```python
from build123d import *

# Parameters (mm, degrees)
ESQUISSE1_W             = 54.1
ESQUISSE1_H             = 54.4
BOSS_EXTRU_1_DEPTH      = 19
ESQUISSE2_W             = 20
ESQUISSE2_H             = 12
BOSS_EXTRU_2_DEPTH      = 15
ESQUISSE3_W             = 9
ESQUISSE3_H             = 18
BOSS_EXTRU_3_DEPTH      = 5
ESQUISSE4_R             = 1.5
ENL_V_MAT_EXTRU_1_DEPTH = 81.387623426


with BuildPart() as part:
    # Esquisse1 → Boss.-Extru.1 (new body)
    with BuildSketch(Plane(origin=(0, 0, 0), x_dir=(1, 0, 0), z_dir=(0, 1, 0))):
        with Locations((27.05, 27.2)):
            Rectangle(ESQUISSE1_W, ESQUISSE1_H)
    extrude(amount=BOSS_EXTRU_1_DEPTH)

    # Esquisse2 → Boss.-Extru.2 (add)
    with BuildSketch(Plane.XZ):
        with Locations((27, -28.4)):
            Rectangle(ESQUISSE2_W, ESQUISSE2_H)
    extrude(amount=BOSS_EXTRU_2_DEPTH)

    # Esquisse3 → Boss.-Extru.3 (add)
    with BuildSketch(Plane(origin=(0, 19, 0), x_dir=(1, 0, 0), z_dir=(0, 1, 0))):
        with Locations((46.6, 43.9)):
            Rectangle(ESQUISSE3_W, ESQUISSE3_H)
        with Locations((7.5, 11)):
            Rectangle(ESQUISSE3_W, ESQUISSE3_H)
    extrude(amount=BOSS_EXTRU_3_DEPTH)

    # Esquisse4 → Enlèv. mat.-Extru.1 (cut, through all)
    with BuildSketch(Plane.XZ):
        with Locations(Location((50.1, -30, 0), (0, 0, 270))):
            Circle(ESQUISSE4_R)
    extrude(amount=-ENL_V_MAT_EXTRU_1_DEPTH, mode=Mode.SUBTRACT)


solid = part.part
```
Model file for the job. Use its own axes, mm. A direction names the side the tool comes from. Give positions to 0.01 mm unless a question says otherwise; leave off trailing zeros. Write each loop counter-clockwise with the first axis right and the second up, starting at its lowest first coordinate (ties: lowest second). Pieces come first, ordered by that corner, then holes. Notation, with made-up numbers: M 25.25,-3 L 66.25,-3 A20 ccw 66.25,11 Z; hole C 84,55 d3. An arc over 180 degrees is marked long. Use a Markdown table: item, result.
1) Pin check, flat tips, straight feed: pin 1 (5.5 mm diameter, centred on x = 45.5, y = 22, fed in from +Z); pin 2 (1.5 mm diameter, centred on x = 7.5, y = 22.5, fed in from +Z); pin 3 (1 mm diameter, centred on x = 35, z = -7, fed in from +Y). Stop position of each tip, or through.
Responses:
| item | result |
|---|---|
| pin 1 | stops at z = -34.9 |
| pin 2 | stops at z = -2 |
| pin 3 | stops at y = 19 |
2) Cut at B-B (z = -30). List the corners of the cut face in (x, y).
Responses:
| item | result |
|---|---|
| outline | M 0,0 L 17,0 L 17,-15 L 37,-15 L 37,0 L 48.6,0 L 48.6,19 L 0,19 Z; M 51.6,0 L 54.1,0 L 54.1,19 L 51.6,19 Z |
3) Cut at A-A (x = 50.1). List the corners of the cut face in (y, z), and give its area (3 significant figures).
Responses:
| item | result |
|---|---|
| outline | M 0,-54.4 L 19,-54.4 L 19,-52.9 L 24,-52.9 L 24,-34.9 L 19,-34.9 L 19,-31.5 L 0,-31.5 Z; M 0,-28.5 L 19,-28.5 L 19,0 L 0,0 Z |
| area | 1,070 mm2 |
4) Cut at C-C (x = 23.5). List the corners of the cut face in (y, z).
Responses:
| item | result |
|---|---|
| outline | M -15,-34.4 L 0,-34.4 L 0,-54.4 L 19,-54.4 L 19,0 L 0,0 L 0,-22.4 L -15,-22.4 Z |
5) Pull direction X, two halves, no side cores. Call faces 1 (the flat face through (54.1, 9, -27)), 2 (the flat face through (17, -7, -28)), 3 (the cylindrical face through (51.11, 9.37, -28.89)), 4 (the flat face through (27, 9, 0)): +X half, -X half, draft (parallel to the pull), parting line (faces both ways), or undercut.
Responses:
| item | result |
|---|---|
| face 1 | +X half |
| face 2 | -X half |
| face 3 | undercut |
| face 4 | draft |
6) Drill centre lines: line 1 (X direction, y = 4, z = -30); line 2 (Y direction, x = 6.5, z = -13); line 3 (Y direction, x = 11, z = -42). Where is each one in solid material? Low to high. Write a range as from..to.
Responses:
| item | result |
|---|---|
| line 1 | x = 0..48.6, 51.6..54.1 |
| line 2 | y = 0..24 |
| line 3 | y = 0..19 |
7) Cut at D-D (z = -42). List the corners of the cut face in (x, y).
Responses:
| item | result |
|---|---|
| outline | M 0,0 L 54.1,0 L 54.1,19 L 51.1,19 L 51.1,24 L 42.1,24 L 42.1,19 L 0,19 Z |
8) Tool access for faces 5 (the flat face through (7, 21, -2)), 6 (the flat face through (12, 21, -11)), 7 (the flat face through (7, 21, -20)), 8 (the flat face through (3, 21, -11)): list every direction of +Z, -Z, +X, -X, +Y, -Y with a clear straight run to the whole face (end or side of a thin tool).
Responses:
| item | result |
|---|---|
| face 5 | +Z, +X, -X, +Y |
| face 6 | +Z, -Z, +X, +Y |
| face 7 | -Z, +X, -X, +Y |
| face 8 | +Z, -Z, -X, +Y |
